from build123d import *

# Parameters (mm, degrees)
SKETCH1_W           = 35.5
SKETCH1_H           = 22.5
BOSS_EXTRUDE1_DEPTH = 3.6
SKETCH2_W           = 15.8
SKETCH2_H           = 4
BOSS_EXTRUDE2_DEPTH = 4.7
SKETCH3_R           = 6.5
BOSS_EXTRUDE3_DEPTH = 24.6
SKETCH4_W           = 6
SKETCH4_H           = 7.5
CUT_EXTRUDE1_DEPTH  = 16
SKETCH5_W           = 1
SKETCH5_H           = 0.4
SKETCH5_W_2         = 0.4
SKETCH5_H_2         = 1
BOSS_EXTRUDE4_DEPTH = 16
FILLET1_R           = 1
FILLET2_R           = 1.75
BOSS_EXTRUDE5_DEPTH = 0.4
SKETCH7_W           = 1.8
SKETCH7_H           = 5.4
BOSS_EXTRUDE6_DEPTH = 26
FILLET3_R           = 0.75


with BuildPart() as part:
    # Sketch1 → Boss-Extrude1 (new body)
    with BuildSketch(Plane(origin=(0, 0, 0), x_dir=(0, 1, 0), z_dir=(0, 0, 1))):
        Rectangle(SKETCH1_W, SKETCH1_H)
    extrude(amount=BOSS_EXTRUDE1_DEPTH)

    # Sketch2 → Boss-Extrude2 (add)
    with BuildSketch(Plane.XY.offset(3.6)):
        Rectangle(SKETCH2_W, SKETCH2_H)
    extrude(amount=BOSS_EXTRUDE2_DEPTH)

    # Sketch3 → Boss-Extrude3 (add)
    with BuildSketch(Plane(origin=(0, 0, 0), x_dir=(1, 0, 0), z_dir=(0, 0, -1))):
        Circle(SKETCH3_R)
    extrude(amount=BOSS_EXTRUDE3_DEPTH)

    # Sketch4 → Cut-Extrude1 (cut)
    with BuildSketch(Plane(origin=(0, 0, -24.6), x_dir=(1, 0, 0), z_dir=(0, 0, -1))):
        Rectangle(SKETCH4_W, SKETCH4_H)
    extrude(amount=-CUT_EXTRUDE1_DEPTH, mode=Mode.SUBTRACT)

    # Sketch5 → Boss-Extrude4 (add)
    with BuildSketch(Plane(origin=(0, 0, -24.6), x_dir=(-1, 0, 0), z_dir=(0, 0, -1))):
        with Locations((0, 3.75)):
            Rectangle(SKETCH5_W, SKETCH5_H)
        with Locations((-3, 0)):
            Rectangle(SKETCH5_W_2, SKETCH5_H_2)
        with Locations((0, -3.75)):
            Rectangle(SKETCH5_W, SKETCH5_H)
        with Locations((3, 0)):
            Rectangle(SKETCH5_W_2, SKETCH5_H_2)
    extrude(amount=-BOSS_EXTRUDE4_DEPTH)

    # Fillet1
    fillet1_edges = [part.edges().sort_by_distance(p)[0] for p in [
        (11.25, 17.75, 1.8),
        (11.25, -17.75, 1.8),
        (-11.25, -17.75, 1.8),
        (-11.25, 17.75, 1.8),
    ]]
    fillet(fillet1_edges, radius=FILLET1_R)

    # Fillet2
    fillet2_edges = [part.edges().sort_by_distance(p)[0] for p in [
        (7.9, -2, 5.95),
        (7.9, 2, 5.95),
        (-7.9, 2, 5.95),
        (-7.9, -2, 5.95),
        (7.9, 0, 8.3),
        (0, 2, 8.3),
        (-7.9, 0, 8.3),
        (0, -2, 8.3),
    ]]
    fillet(fillet2_edges, radius=FILLET2_R)

    # Sketch6 → Boss-Extrude5 (add)
    with BuildSketch(Plane.XY.offset(3.6)):
        Polygon((3.5, 2.75), (-3.5, 2.75), (0, 6.25), align=None)
        Polygon((3.5, -2.75), (-3.5, -2.75), (0, -6.25), align=None)
    extrude(amount=BOSS_EXTRUDE5_DEPTH)

    # Sketch7 → Boss-Extrude6 (add)
    with BuildSketch(Plane(origin=(0, 0, -24.6), x_dir=(1, 0, 0), z_dir=(0, 0, -1))):
        with Locations((0, 6.5)):
            Rectangle(SKETCH7_W, SKETCH7_H)
        with Locations((0, -6.5)):
            Rectangle(SKETCH7_W, SKETCH7_H)
    extrude(amount=-BOSS_EXTRUDE6_DEPTH)

    # Fillet3
    fillet3_edges = [part.edges().sort_by_distance(p)[0] for p in [
        (0.9, -9.2, -12.3),
        (-0.9, -9.2, -12.3),
        (0.9, 9.2, -12.3),
        (-0.9, 9.2, -12.3),
    ]]
    fillet(fillet3_edges, radius=FILLET3_R)


solid = part.part
CAD build for the part. Positions are in the model's coordinates, mm. A direction names the side the tool comes from. Round coordinates to 2 decimals unless told otherwise and drop trailing zeros. Loops run counter-clockwise (first coordinate to the right, second up) from the corner with the lowest first, then second, coordinate; pieces in that order, holes last.
(1) Cut at C-C (x = 4.5). Give the cut face in (y, z).
(2) Which spindle directions (+Z, -Z, +X, -X, +Y, -Y) get a long thin tool onto all of the face, cutting with end or side? Do faces 5 (the flat face through (-5.2, -4.2, 0)), 6 (the flat face through (0, -4, 4)), 7 (the flat face through (-1.77, 4.48, 3.8)). Say none if no direction does.
(3) Drop flat-ended pins along their axis: pin 1 (2 mm diameter, centred on x = -2, z = -20.5, fed in from +Y); pin 2 (12 mm diameter, centred on x = 1, z = -18, fed in from +Y); pin 3 (3.5 mm diameter, centred on y = 3, z = -15, fed in from -X); pin 4 (1.5 mm diameter, centred on x = -6.5, y = 1, fed in from +Z). Give the stop position or say it passes through.
(4) Cut at B-B (z = -3). Give the cut face in (x, y), plus the area to 3 significant figures.
(5) Two-plate mould, pull along Y, no slides. Class faces 1 (the cylindrical face through (-10.949, -17.465, 1.825)), 2 (the flat face through (-0.9, -7, -12)), 3 (the flat face through (2.8, 0, -17)), 4 (the cylindrical face through (7.401, 1.474, 5.096)): +Y half, -Y half, draft (parallel to the pull), parting line (faces both ways), or undercut.
(6) Wall check: line 1 along Z through (x, y) = (0.5, 15); line 2 along Y through (x, z) = (1, -11); line 3 along Z through (x, y) = (-1.5, 5). Give the ranges that are in metal, low to high.
(7) Cut at D-D (y = 5). Give the cut face in (x, z).
Findings below:
1. outline: (-17.75, 0) - (-4.69, 0) - (-4.69, -24.6) - (4.69, -24.6) - (4.69, 0) - (17.75, 0) - (17.75, 3.6) - (2, 3.6) - (2, 6.55) arc R1.75 ccw to (0.25, 8.3) - (-0.25, 8.3) arc R1.75 ccw to (-2, 6.55) - (-2, 3.6) - (-17.75, 3.6) - close
2. face 5: -Z
2. face 6: +Z, +X, -X, -Y
2. face 7: +Z, -X, +Y
3. pin 1: stops at y = 6.42
3. pin 2: stops at y = 9.2
3. pin 3: stops at x = -6.38
3. pin 4: stops at z = 8.3
4. outline: (-0.9, -8.45) arc R0.75 ccw to (-0.15, -9.2) - (0.15, -9.2) arc R0.75 ccw to (0.9, -8.45) - (0.9, -6.44) arc R6.5 ccw to (0.9, 6.44) - (0.9, 8.45) arc R0.75 ccw to (0.15, 9.2) - (-0.15, 9.2) arc R0.75 ccw to (-0.9, 8.45) - (-0.9, 6.44) arc R6.5 ccw to (-0.9, -6.44) - close
4. area: 142 mm2
5. face 1: -Y half
5. face 2: draft
5. face 3: undercut
5. face 4: +Y half
6. line 1: z = 0 to 3.6
6. line 2: y = -6.42 to -3.75, 3.75 to 6.42
6. line 3: z = -24.6 to 3.6
7. outline: (-11.25, 0) - (-4.15, 0) - (-4.15, -24.6) - (4.15, -24.6) - (4.15, 0) - (11.25, 0) - (11.25, 3.6) - (1.25, 3.6) - (1.25, 4) - (-1.25, 4) - (-1.25, 3.6) - (-11.25, 3.6) - close
